Read the model definition and answer for the solid it produces. Units are mm, in the model's axes. Face numbers are marked on the shaded views. A direction names the side the tool comes from. Coordinates: 2 decimals unless noted, no trailing zeros. Order: outer loops, then holes, each group sorted by start corner. A loop starts at its lowest first (then second) coordinate and runs counter-clockwise, first axis right, second up. Notation, with made-up numbers: M -26,-30 L 28,-30 A18 cw 28,-5 Z; hole C -24.5,-24 d6. An arc over 180 degrees is marked long. Write each question's results on one line, items separated by ' | '.
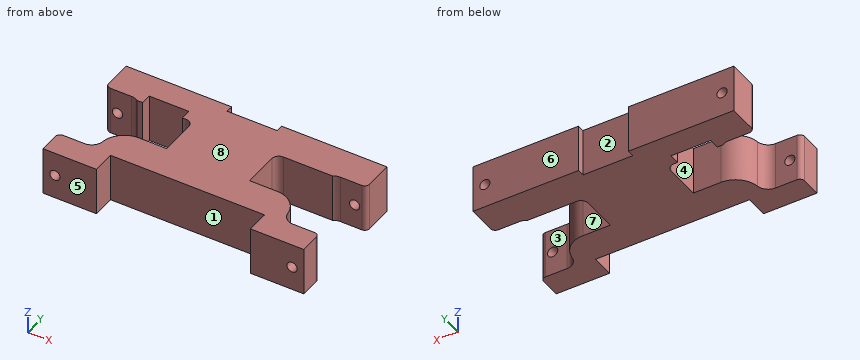
```python
from build123d import *

# Parameters (mm, degrees)
SKETCH1_W                = 110
SKETCH1_H                = 20.25
SKETCH1_R                = 2.159
BOSS_EXTRUDE1_DEPTH      = 43.175
CUT_EXTRUDE3_START       = 39
SKETCH2_W                = 74.945935845
SKETCH2_H                = 32
CUT_EXTRUDE3_DEPTH       = 17
CUT_EXTRUDE4_START       = -39
SKETCH2_3_W              = 74.945935845
SKETCH2_3_H              = 32
CUT_EXTRUDE4_DEPTH       = 17
FILLET1_R                = 5
FILLET2_R                = 2
SKETCH10_W               = 65
SKETCH10_H               = 20.25
CUT_EXTRUDE8_DEPTH       = 3.175
SKETCH11_W               = 30
SKETCH11_H               = 18
SKETCH11_W_2             = 29.367311722
CUT_EXTRUDE9_DEPTH       = 21.25
FILLET3_R                = 10
FILLET5_R                = 3
SKETCH16_W               = 22.5
SKETCH16_H               = 20.25
BOSS_EXTRUDE4_DEPTH      = 6.35
SKETCH13_W               = 110
SKETCH13_H               = 20.25
BOSS_EXTRUDE5_DEPTH      = 3.675
SKETCH19_W               = 44.5
SKETCH19_H               = 20.25
BOSS_EXTRUDE6_DEPTH      = 3
SKETCH20_R               = 2.159
CUT_EXTRUDE10_DEPTH      = 46.8500001
CUT_EXTRUDE10_DEPTH_BACK = 11.3500001
SKETCH21_W               = 16.684617085
SKETCH21_H               = 4.437831476
CUT_EXTRUDE11_DEPTH      = 21.2500001


with BuildPart() as part:
    # Sketch1 → Boss-Extrude1 (new body)
    with BuildSketch(Plane(origin=(0, 0, 0), x_dir=(1, 0, 0), z_dir=(0, 1, 0))):
        Rectangle(SKETCH1_W, SKETCH1_H)
        with Locations((-50, 0)):
            Circle(SKETCH1_R, mode=Mode.SUBTRACT)
        with Locations((50, 0)):
            Circle(SKETCH1_R, mode=Mode.SUBTRACT)
    extrude(amount=BOSS_EXTRUDE1_DEPTH)

    # Sketch2 → Cut-Extrude3 (cut, through all)
    with BuildSketch(Plane(origin=(0, 0, 0), x_dir=(0, 0, -1), z_dir=(1, 0, 0)).offset(CUT_EXTRUDE3_START)):
        with Locations((0.587900532, 20)):
            Rectangle(SKETCH2_W, SKETCH2_H)
    extrude(amount=CUT_EXTRUDE3_DEPTH, mode=Mode.SUBTRACT)

    # Sketch2_3 → Cut-Extrude4 (cut, through all)
    with BuildSketch(Plane(origin=(0, 0, 0), x_dir=(0, 0, -1), z_dir=(1, 0, 0)).offset(CUT_EXTRUDE4_START)):
        with Locations((0.587900532, 20)):
            Rectangle(SKETCH2_3_W, SKETCH2_3_H)
    extrude(amount=-CUT_EXTRUDE4_DEPTH, mode=Mode.SUBTRACT)

    # Fillet1
    fillet1_edges = [part.edges().sort_by_distance(p)[0] for p in [
        (39, 36, 0),
        (39, 4, 0),
        (-39, 4, 0),
        (-39, 36, 0),
    ]]
    fillet(fillet1_edges, radius=FILLET1_R)

    # Fillet2
    fillet2_edges = [part.edges().sort_by_distance(p)[0] for p in [
        (55, 4, 0),
        (55, 36, 0),
        (-55, 36, 0),
        (-55, 4, 0),
    ]]
    fillet(fillet2_edges, radius=FILLET2_R)

    # Sketch10 → Cut-Extrude8 (cut)
    with BuildSketch(Plane.XZ):
        Rectangle(SKETCH10_W, SKETCH10_H)
    extrude(amount=-CUT_EXTRUDE8_DEPTH, mode=Mode.SUBTRACT)

    # Sketch11 → Cut-Extrude9 (cut, through all)
    with BuildSketch(Plane.XY.offset(10.125)):
        with Locations((32.5, 26.096159603)):
            Rectangle(SKETCH11_W, SKETCH11_H)
        with Locations((-32.183655861, 26.096159603)):
            Rectangle(SKETCH11_W_2, SKETCH11_H)
    extrude(amount=-CUT_EXTRUDE9_DEPTH, mode=Mode.SUBTRACT)

    # Fillet3
    fillet3_edges = [part.edges().sort_by_distance(p)[0] for p in [
        (39, 17.096159603, 0),
        (-39, 17.096159603, 0),
    ]]
    fillet(fillet3_edges, radius=FILLET3_R)

    # Fillet5
    fillet5_edges = [part.edges().sort_by_distance(p)[0] for p in [
        (-17.5, 35.096159603, 0),
        (17.5, 35.096159603, 0),
    ]]
    fillet(fillet5_edges, radius=FILLET5_R)

    # Sketch16 → Boss-Extrude4 (add)
    with BuildSketch(Plane.XZ):
        with Locations((-43.75, 0)):
            Rectangle(SKETCH16_W, SKETCH16_H)
        with Locations((43.75, 0)):
            Rectangle(SKETCH16_W, SKETCH16_H)
    extrude(amount=BOSS_EXTRUDE4_DEPTH)

    # Sketch13 → Boss-Extrude5 (add)
    with BuildSketch(Plane(origin=(0, 43.175, 0), x_dir=(1, 0, 0), z_dir=(0, 1, 0))):
        Rectangle(SKETCH13_W, SKETCH13_H)
    extrude(amount=BOSS_EXTRUDE5_DEPTH)

    # Sketch19 → Boss-Extrude6 (add)
    with BuildSketch(Plane(origin=(0, 46.85, 0), x_dir=(1, 0, 0), z_dir=(0, 1, 0))):
        with Locations((-32.75, 0)):
            Rectangle(SKETCH19_W, SKETCH19_H)
        with Locations((32.75, 0)):
            Rectangle(SKETCH19_W, SKETCH19_H)
    extrude(amount=BOSS_EXTRUDE6_DEPTH)

    # Sketch20 → Cut-Extrude10 (cut, two sides)
    with BuildSketch(Plane(origin=(0, 4, 0), x_dir=(1, 0, 0), z_dir=(0, 1, 0))) as cut_extrude10_sk:
        with Locations((-50, 0)):
            Circle(SKETCH20_R)
        with Locations((50, 0)):
            Circle(SKETCH20_R)
    extrude(amount=CUT_EXTRUDE10_DEPTH, mode=Mode.SUBTRACT)
    extrude(cut_extrude10_sk.sketch, amount=-CUT_EXTRUDE10_DEPTH_BACK, mode=Mode.SUBTRACT)

    # Sketch21 → Cut-Extrude11 (cut, through all)
    with BuildSketch(Plane.XY.offset(10.125)):
        with Locations((-30.45912654, 37.315075341)):
            Rectangle(SKETCH21_W, SKETCH21_H)
    extrude(amount=-CUT_EXTRUDE11_DEPTH, mode=Mode.SUBTRACT)


solid = part.part
```
(1) For the marked faces 1, 2, 3 and 4, determine the directions among +Z, -Z, +X, -X, +Y, -Y from which every point of the face is accessible in a straight line to the end or side of a thin tool.
Conclusion:
face 1: +Z, -Z, -Y | face 2: +Z, -Z, +Y | face 3: +Z, -Z, +X | face 4: +Z, -Z, -X
(2) The mould has two halves that part along Y. Classify the marked faces 5, 6, 7 and 8: pulls with the +Y half, pulls with the -Y half, needs draft (parallel to the pull), parting line crosses it, or undercut.
Conclusion:
face 5: pulls with the -Y half | face 6: pulls with the +Y half | face 7: undercut | face 8: needs draft
(3) The part is cut by section A-A, the plane x = -50. Write down the section's boundary in (y, z) (3 decimals).
Conclusion:
outline: M -6.35,-10.125 L 4,-10.125 L 4,-2.159 L -6.35,-2.159 Z; M -6.35,2.159 L 4,2.159 L 4,10.125 L -6.35,10.125 Z; M 36,-10.125 L 49.85,-10.125 L 49.85,-2.159 L 36,-2.159 Z; M 36,2.159 L 49.85,2.159 L 49.85,10.125 L 36,10.125 Z
(4) Given pin 1 (10 mm diameter, centred on y = 16.5, z = -5, fed in from -X); pin 2 (1.8 mm diameter, centred on x = -21, z = 1.5, fed in from -Y) (3 decimals); pin 3 (3 mm diameter, centred on y = 20, z = -0.5, fed in from -X), each flat-ended and moving along its own axis, determine where each tip first touches the part or whether it passes through.
Conclusion:
pin 1: x = -38.1 | pin 2: y = 3.175 | pin 3: x = -17.5
(5) The part is cut by section B-B, the plane x = 5. Write down the section's boundary in (y, z) (3 decimals).
Conclusion:
outline: M 3.175,-10.125 L 46.85,-10.125 L 46.85,10.125 L 3.175,10.125 Z
(6) Straight lines are drawn through the part: line 1 (Y direction, x = 29.5, z = 0.75) (3 decimals); line 2 (X direction, y = 2.6, z = 0); line 3 (X direction, y = -2, z = 0). For each, find the intervals that lie inside material, in ascending order.
Conclusion:
line 1: 3.175 to 17.089, 35.096 to 49.85 | line 2: -54.91 to -52.16, -47.84 to -32.5, 32.5 to 47.84, 52.16 to 54.91 | line 3: -55 to -52.16, -47.84 to -32.5, 32.5 to 47.84, 52.16 to 55
